Read the model definition and answer for the solid it produces. Units are mm, in the model's axes. Face numbers are marked on the shaded views. Round coordinates to 2 decimals unless told otherwise and drop trailing zeros. Write each loop counter-clockwise with the first axis right and the second up, starting at its lowest first coordinate (ties: lowest second). Pieces come first, ordered by that corner, then holes. Notation, with made-up numbers: M -25.5,22.25 L -12.5,22.25 A15 ccw -12.5,32.25 Z; hole C -27.5,65 d6. An arc over 180 degrees is marked long. Use one line per item in the form item = value. Start each with the question number.
```python
from build123d import *

# Parameters (mm, degrees)
F1_DEPTH   = 12.7
F4_D       = 4.4958
F4_ON_F3_D = 4.4958


with BuildPart() as f1:
    # F0 (on Front) → F1 (new body)
    with BuildSketch(Plane.XZ):
        with BuildLine():
            Line((-51.8633585078, -3.48165389), (-51.8633585078, -35.23165389))
            Line((-51.8633585078, -35.23165389), (-43.9258585078, -35.23165389))
            ThreePointArc((-43.9258585078, -35.23165389), (-42.3383585078, -33.64415389), (-40.7508585078, -35.23165389))
            Line((-40.7508585078, -35.23165389), (-34.4008585078, -35.23165389))
            ThreePointArc((-34.4008585078, -35.23165389), (-32.8133585078, -33.64415389), (-31.2258585078, -35.23165389))
            Line((-31.2258585078, -35.23165389), (-24.8631585078, -35.23165389))
            ThreePointArc((-24.8631585078, -35.23165389), (-21.6881585078, -32.05665389), (-18.5131585078, -35.23165389))
            Line((-18.5131585078, -35.23165389), (-12.5060585078, -35.23165389))
            ThreePointArc((-12.5060585078, -35.23165389), (-10.9185585078, -33.64415389), (-9.3310585078, -35.23165389))
            Line((-9.3310585078, -35.23165389), (-1.4189585078, -35.23165389))
            Line((-1.4189585078, -35.23165389), (-1.4189585078, -3.48165389))
            Line((-1.4189585078, -3.48165389), (-51.8633585078, -3.48165389))
        make_face()
    extrude(amount=F1_DEPTH)

    # F4 (through all)
    with Locations(Plane(origin=(0, 0, -35.23165389), x_dir=(1, 0, 0), z_dir=(0, 0, -1))):
        with Locations((-48.6883585078, 6.35)):
            Hole(F4_D / 2)

    # F4 on F3 (through all)
    with Locations(Plane(origin=(0, 0, -35.23165389), x_dir=(1, 0, 0), z_dir=(0, 0, -1))):
        with Locations((-4.5939585078, 6.35)):
            Hole(F4_ON_F3_D / 2)


solid = f1.part
```
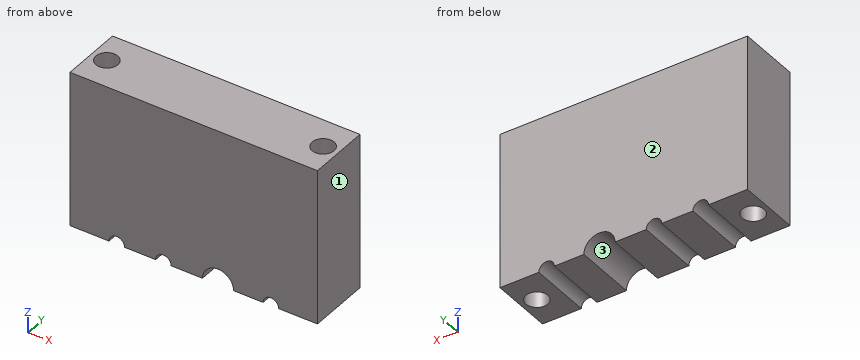
Q1. Find section B-B on z = -12.5. Write down the section's boundary in (x, y).
Q2. Find section A-A on y = -6.35. Count the separate pieces of the cut face and the enclosed holes in it, and give its area (3 significant figures).
Q3. For a pull along X with two mould halves and no side action, classify the marked faces 1, 2 and 3 as +X half, -X half, draft (parallel to the pull), parting line (faces both ways), or undercut.
Q4. Straight lines are drawn through the part: line 1 (X direction, y = -7.75, z = -16); line 2 (Y direction, x = -49, z = -26); line 3 (Y direction, x = -5.5, z = -11.5). For each, find the intervals that lie inside material, in ascending order. Write a range as [from, to].
Q5. Find section D-D on z = -33. Write down the section's boundary in (x, y), and give its area (3 significant figures).
Response:
q1.outline = M -51.86,-12.7 L -1.42,-12.7 L -1.42,0 L -51.86,0 Z; hole C -48.69,-6.35 d4.5; hole C -4.59,-6.35 d4.5
q2.separate_pieces = 3
q2.enclosed_holes = 0
q2.area = 1,290 mm²
q3.face_1 = +X half
q3.face_2 = draft
q3.face_3 = undercut
q4.line_1 = [-51.86, -50.45], [-46.93, -6.35], [-2.84, -1.42]
q4.line_2 = [-12.7, -8.58], [-4.12, 0]
q4.line_3 = [-12.7, -8.41], [-4.29, 0]
q5.outline = M -51.86,-12.7 L -23.95,-12.7 L -23.95,0 L -51.86,0 Z; M -19.43,-12.7 L -1.42,-12.7 L -1.42,0 L -19.43,0 Z; hole C -48.69,-6.35 d4.5; hole C -4.59,-6.35 d4.5
q5.area = 552 mm²
